from build123d import *

# Parameters (mm, degrees)
BOSS_EXTRUDE1_DEPTH = 20
BOSS_EXTRUDE2_DEPTH = 2.5
BOSS_EXTRUDE3_DEPTH = 2.5
SKETCH4_R           = 2
CUT_EXTRUDE1_DEPTH  = 55.083269132
SKETCH6_R           = 3.1
CUT_EXTRUDE2_DEPTH  = 56.587768439
FILLET1_R           = 2
FILLET2_R           = 0.5


with BuildPart() as part:
    # Sketch1 → Boss-Extrude1 (new body)
    with BuildSketch(Plane.XY):
        Polygon((0, 43), (0, 0), (29, 0), (29, 3), (3, 3), (3, 43), align=None)
    extrude(amount=BOSS_EXTRUDE1_DEPTH)

    # Sketch2 → Boss-Extrude2 (add)
    with BuildSketch(Plane.XY.offset(20)):
        Polygon((3, 43), (29, 3), (3, 3), align=None)
    extrude(amount=-BOSS_EXTRUDE2_DEPTH)

    # Sketch3 → Boss-Extrude3 (add)
    with BuildSketch(Plane(origin=(0, 0, 0), x_dir=(-1, 0, 0), z_dir=(0, 0, -1))):
        Polygon((-3, 43), (-29, 3), (-3, 3), align=None)
    extrude(amount=-BOSS_EXTRUDE3_DEPTH)

    # Sketch4 → Cut-Extrude1 (cut, through all)
    with BuildSketch(Plane(origin=(3, 0, 0), x_dir=(0, 0, -1), z_dir=(1, 0, 0))):
        with Locations(Location((-10, 33, 0), (0, 0, 90))):
            Circle(SKETCH4_R)
        with Locations(Location((-10, 13, 0), (0, 0, 90))):
            Circle(SKETCH4_R)
    extrude(amount=-CUT_EXTRUDE1_DEPTH, mode=Mode.SUBTRACT)

    # Sketch6 → Cut-Extrude2 (cut, through all)
    with BuildSketch(Plane.XZ):
        with Locations(Location((19, 10, 0), (0, 0, 270))):
            Circle(SKETCH6_R)
    extrude(amount=-CUT_EXTRUDE2_DEPTH, mode=Mode.SUBTRACT)

    # Fillet1
    fillet1_edges = [part.edges().sort_by_distance(p)[0] for p in [
        (29, 0, 10),
        (3, 3, 10),
        (3, 23, 17.5),
        (16, 3, 17.5),
        (3, 23, 2.5),
        (16, 3, 2.5),
    ]]
    fillet(fillet1_edges, radius=FILLET1_R)

    # Fillet2
    fillet2_edges = [part.edges().sort_by_distance(p)[0] for p in [
        (3, 31, 10),
        (3, 11, 10),
        (19, 3, 13.1),
    ]]
    fillet(fillet2_edges, radius=FILLET2_R)


solid = part.part
Input: part model. Units: mm. Frame: model coordinates. A direction names the side the tool comes from. Give positions to 0.01 mm unless a question says otherwise; leave off trailing zeros. Write each loop counter-clockwise with the first axis right and the second up, starting at its lowest first coordinate (ties: lowest second). Pieces come first, ordered by that corner, then holes.
Q1. Set-up query: faces 1 (the face through (1.268, 11.526, 11.352)), 2 (the face through (15, 3, 10)). Return all of +Z, -Z, +X, -X, +Y, -Y with unobstructed straight access to the full face (end or side cutting, diameter ignored); none if empty.
Q2. Section B-B, the plane z = 10. Output: boundary loops of the cut face in (x, y), plus the area to 3 significant figures.
Q3. Section D-D, the plane z = 14.5. Output: boundary loops of the cut face in (x, y).
Q4. Pull-direction query (Z, two-part tool) for faces 3 (the face through (0, 22, 10)), 4 (the face through (11, 15, 17.5)), 5 (the face through (16.83, 3.57, 16.9)), 6 (the face through (11, 17, 0)); classes: pulls with the +Z half, pulls with the -Z half, needs draft (parallel to the pull), parting line crosses it, or undercut.
Q5. Section A-A, the plane y = 13. Output: boundary loops of the cut face in (x, z), plus the area to 3 significant figures.
Q6. First-contact query: P1, Ø8, axis at y = 17.5, z = 13, coming from the +X side; P2, Ø5.5, axis at y = 18.5, z = 12, coming from the +X side; P3, Ø4.5, axis at y = 13, z = 10, coming from the +X side. Flat tips, straight axial feed; report the tip coordinate or a pass-through.
Q7. Section C-C, the plane x = 19. Output: boundary loops of the cut face in (y, z), plus the area to 3 significant figures.
Q8. Material intervals for probe 1 along Z at (x, y) = (0.85, 33); probe 2 along Z at (x, y) = (15, 15); probe 3 along X at (y, z) = (33.5, 15.5), sorted ascending.
Filled in:
1. face 1: +X, -X
1. face 2: +X, +Y
2. outline: (0, 0) - (15.9, 0) - (15.9, 2.5) arc R0.5 ccw to (15.4, 3) - (5, 3) arc R2 cw to (3, 5) - (3, 10.5) arc R0.5 ccw to (2.5, 11) - (0, 11) - close; (0, 15) - (2.5, 15) arc R0.5 ccw to (3, 15.5) - (3, 30.5) arc R0.5 ccw to (2.5, 31) - (0, 31) - close; (0, 35) - (2.5, 35) arc R0.5 ccw to (3, 35.5) - (3, 43) - (0, 43) - close; (22.1, 0) - (27, 0) arc R2 ccw to (29, 2) - (29, 3) - (22.6, 3) arc R0.5 ccw to (22.1, 2.5) - close
2. area: 164 mm2
3. outline: (0, 0) - (27, 0) arc R2 ccw to (29, 2) - (29, 3) - (5, 3) arc R2 cw to (3, 5) - (3, 43) - (0, 43) - close
4. face 3: needs draft
4. face 4: undercut
4. face 5: undercut
4. face 6: pulls with the -Z half
5. outline: (0, 0) - (22.5, 0) - (22.5, 2.5) - (5, 2.5) arc R2 cw to (3, 4.5) - (3, 7.5) arc R0.5 ccw to (2.5, 8) - (0, 8) - close; (0, 12) - (2.5, 12) arc R0.5 ccw to (3, 12.5) - (3, 15.5) arc R2 cw to (5, 17.5) - (22.5, 17.5) - (22.5, 20) - (0, 20) - close
5. area: 147 mm2
6. P1: stops at x = 3.68
6. P2: stops at x = 3
6. P3: stops at x = 2.93
7. outline: (0, 0) - (18.38, 0) - (18.38, 2.5) - (5, 2.5) arc R2 cw to (3, 4.5) - (3, 6.4) arc R0.5 ccw to (2.5, 6.9) - (0, 6.9) - close; (0, 13.1) - (2.5, 13.1) arc R0.5 ccw to (3, 13.6) - (3, 15.5) arc R2 cw to (5, 17.5) - (18.38, 17.5) - (18.38, 20) - (0, 20) - close
7. area: 120 mm2
8. probe 1: z = 0 to 8, 12 to 20
8. probe 2: z = 0 to 2.5, 17.5 to 20
8. probe 3: x = 0 to 3
